```python
from build123d import *

# Parameters (mm, degrees)
SKETCH1_R           = 2.499995
SKETCH1_R_2         = 2.5
SKETCH1_R_3         = 14.2875
BOSS_EXTRUDE1_DEPTH = 3.175


with BuildPart() as part:
    # Sketch1 → Boss-Extrude1 (new body)
    with BuildSketch(Plane(origin=(1.5875, 0, 0), x_dir=(0, 0, -1), z_dir=(1, 0, 0))):
        with BuildLine():
            Line((54.345399121, 12.19455323), (-13.718855966, 32.143669532))
            ThreePointArc((-13.718855966, 32.143669532), (-18.053428342, 31.606906651), (-20.630025283, 28.080182921))
            Line((-20.630025283, 28.080182921), (-25.733530559, 5.5386286))
            ThreePointArc((-25.733530559, 5.5386286), (-26.673034326, -0.035153342), (-26.9875, -5.678806752))
            Line((-26.9875, -5.678806752), (-26.9875, -314.995580316))
            ThreePointArc((-26.9875, -314.995580316), (-25.942050019, -322.434343457), (-22.886697995, -329.29677646))
            Line((-22.886697995, -329.29677646), (86.89264859, -504.980455375))
            ThreePointArc((86.89264859, -504.980455375), (90.849314805, -507.802717959), (95.642741328, -507.000573458))
            Line((95.642741328, -507.000573458), (111.133848853, -497.320655139))
            ThreePointArc((111.133848853, -497.320655139), (113.473140107, -494.725479093), (114.085519672, -491.285680619))
            Line((114.085519672, -491.285680619), (63.406704813, 1.306972618))
            ThreePointArc((63.406704813, 1.306972618), (60.534946173, 8.131395413), (54.345399121, 12.19455323))
        make_face()
        with Locations(Location((0, -261.947790158, 0), (0, 0, 180))):
            Circle(SKETCH1_R, mode=Mode.SUBTRACT)
        with Locations(Location((0, -141.947790158, 0), (0, 0, 180))):
            Circle(SKETCH1_R, mode=Mode.SUBTRACT)
        with Locations(Location((22.230640813, -39.122879855, 0), (0, 0, 180))):
            Circle(SKETCH1_R, mode=Mode.SUBTRACT)
        with Locations(Location((-13.49375, -44.45, 0), (0, 0, 180))):
            Circle(SKETCH1_R, mode=Mode.SUBTRACT)
        with Locations(Location((41.976634925, -416.065160512, 0), (0, 0, 180))):
            Circle(SKETCH1_R_2, mode=Mode.SUBTRACT)
        with Locations(Location((72.439391351, -397.029917647, 0), (0, 0, 180))):
            Circle(SKETCH1_R_2, mode=Mode.SUBTRACT)
        with Locations(Location((53.404148486, -366.567161221, 0), (0, 0, 180))):
            Circle(SKETCH1_R_2, mode=Mode.SUBTRACT)
        with Locations(Location((22.94139206, -385.602404086, 0), (0, 0, 180))):
            Circle(SKETCH1_R_2, mode=Mode.SUBTRACT)
        with Locations(Location((0, -201.947790158, 0), (0, 0, 180))):
            Circle(SKETCH1_R_2, mode=Mode.SUBTRACT)
        with Locations(Location((61.9125, -233.697790158, 0), (0, 0, 180))):
            Circle(SKETCH1_R_2, mode=Mode.SUBTRACT)
        with Locations(Location((61.9125, -170.197790158, 0), (0, 0, 180))):
            Circle(SKETCH1_R_2, mode=Mode.SUBTRACT)
        with Locations(Location((0, 0, 0), (0, 0, 180))):
            Circle(SKETCH1_R_3, mode=Mode.SUBTRACT)
        with Locations(Location((0, -88.9, 0), (0, 0, 180))):
            Circle(SKETCH1_R_3, mode=Mode.SUBTRACT)
        with Locations(Location((0, -314.995580316, 0), (0, 0, 180))):
            Circle(SKETCH1_R_3, mode=Mode.SUBTRACT)
        with Locations(Location((44.461281626, -78.24575971, 0), (0, 0, 180))):
            Circle(SKETCH1_R_3, mode=Mode.SUBTRACT)
        with Locations(Location((58.629287829, -432.78796896, 0), (0, 0, 180))):
            Circle(SKETCH1_R_2, mode=Mode.SUBTRACT)
        with Locations(Location((65.359262485, -443.558179782, 0), (0, 0, 180))):
            Circle(SKETCH1_R_2, mode=Mode.SUBTRACT)
        with Locations(Location((72.089237141, -454.328390603, 0), (0, 0, 180))):
            Circle(SKETCH1_R_2, mode=Mode.SUBTRACT)
        with Locations(Location((78.819211796, -465.098601424, 0), (0, 0, 180))):
            Circle(SKETCH1_R_2, mode=Mode.SUBTRACT)
        with Locations(Location((85.549186452, -475.868812245, 0), (0, 0, 180))):
            Circle(SKETCH1_R_2, mode=Mode.SUBTRACT)
        with Locations(Location((92.279161108, -486.639023066, 0), (0, 0, 180))):
            Circle(SKETCH1_R_2, mode=Mode.SUBTRACT)
        with Locations(Location((99.009135764, -497.409233887, 0), (0, 0, 180))):
            Circle(SKETCH1_R_2, mode=Mode.SUBTRACT)
        with Locations(Location((-15.265789691, 26.86569681, 0), (0, 0, 180))):
            Circle(SKETCH1_R_2, mode=Mode.SUBTRACT)
        with BuildLine():
            Line((40.695767644, -376.820032614), (41.660262631, -378.363547244))
            ThreePointArc((41.660262631, -378.363547244), (47.191765144, -377.037364423), (52.802303033, -377.974458618))
            Line((52.802303033, -377.974458618), (53.656778421, -376.367424143))
            ThreePointArc((53.656778421, -376.367424143), (56.023511943, -375.64384109), (56.747094996, -378.010574612))
            Line((56.747094996, -378.010574612), (55.892619609, -379.617609087))
            ThreePointArc((55.892619609, -379.617609087), (59.806878879, -383.744939376), (61.800600445, -389.072354815))
            Line((61.800600445, -389.072354815), (63.619570819, -389.008834969))
            ThreePointArc((63.619570819, -389.008834969), (65.429578885, -390.696694798), (63.741719057, -392.506702864))
            Line((63.741719057, -392.506702864), (61.922748683, -392.570222709))
            ThreePointArc((61.922748683, -392.570222709), (60.305505438, -398.023735817), (56.688689115, -402.41405706))
            Line((56.688689115, -402.41405706), (57.653184101, -403.95757169))
            ThreePointArc((57.653184101, -403.95757169), (57.096458646, -406.369014571), (54.685015765, -405.812289115))
            Line((54.685015765, -405.812289115), (53.720520779, -404.268774485))
            ThreePointArc((53.720520779, -404.268774485), (48.189018265, -405.594957305), (42.578480376, -404.65786311))
            Line((42.578480376, -404.65786311), (41.724004989, -406.264897585))
            ThreePointArc((41.724004989, -406.264897585), (39.357271466, -406.988480637), (38.633688414, -404.621747115))
            Line((38.633688414, -404.621747115), (39.488163801, -403.01471264))
            ThreePointArc((39.488163801, -403.01471264), (35.573904532, -398.887382352), (33.580182967, -393.559966914))
            Line((33.580182967, -393.559966914), (31.761212592, -393.623486759))
            ThreePointArc((31.761212592, -393.623486759), (29.951204527, -391.935626932), (31.639064354, -390.125618866))
            Line((31.639064354, -390.125618866), (33.458034728, -390.062099021))
            ThreePointArc((33.458034728, -390.062099021), (35.075277972, -384.608585913), (38.692094295, -380.218264669))
            Line((38.692094295, -380.218264669), (37.727599308, -378.674750039))
            ThreePointArc((37.727599308, -378.674750039), (38.284324764, -376.263307159), (40.695767644, -376.820032614))
        make_face(mode=Mode.SUBTRACT)
        Polygon((45.984288499, -424.534697371), (56.75449932, -417.804722715), (57.284418584, -418.652770811), (46.514207763, -425.382745467), align=None, mode=Mode.SUBTRACT)
        Polygon((65.200065755, -417.450416925), (71.930040411, -428.220627746), (71.081992315, -428.75054701), (64.352017658, -417.980336189), align=None, mode=Mode.SUBTRACT)
    extrude(amount=-BOSS_EXTRUDE1_DEPTH)


solid = part.part
```
Build history of the part. All positions in model axes, mm. Give positions to 0.01 mm unless a question says otherwise; leave off trailing zeros. Loops run counter-clockwise (first coordinate to the right, second up) from the corner with the lowest first, then second, coordinate; pieces in that order, holes last.
Item 1: Slice it at C-C, the plane y = -57. List the corners of the cut face in (x, z).
Answers follow:
outline: (-1.59, -69.41) - (1.59, -69.41) - (1.59, 26.99) - (-1.59, 26.99) - close
Item 2: Slice it at A-A, the plane y = -308. List the corners of the cut face in (x, z).
Answers follow:
outline: (-1.59, -95.23) - (1.59, -95.23) - (1.59, -12.46) - (-1.59, -12.46) - close; (-1.59, 12.46) - (1.59, 12.46) - (1.59, 26.99) - (-1.59, 26.99) - close
Item 3: Pull direction Z, two halves, no side cores. Call faces 1 (the face through (0.022, -0.628, -14.274)), 2 (the face through (0.022, -415.909, -31.235)), 3 (the face through (0.02, 22.03, -20.79)): released by +Z, released by -Z, zero draft, split by the parting line, or undercut.
Answers follow:
face 1: undercut
face 2: released by +Z
face 3: released by -Z
Item 4: Drill centre lines: line 1 (Y direction, x = -0.1, z = -45.5); line 2 (Y direction, x = 0.9, z = -3); line 3 (Y direction, x = 1.4, z = -35). Where is each one in solid material? Low to high.
Answers follow:
line 1: y = -438.74 to -405.43, -377.2 to -92.5, -64 to 14.79
line 2: y = -370.72 to -328.96, -301.03 to -102.87, -74.93 to -13.97, 13.97 to 27.24
line 3: y = -421.93 to -397.88, -384.75 to -88.95, -67.54 to 17.86
Item 5: Slice it at B-B, the plane x = -1.05. Give the number of separate pieces and of enclosed holes in the cut face, and give its area (3 significant figures).
Answers follow:
separate pieces: 1
enclosed holes: 26
area: 46,600 mm2
